from build123d import *

# Parameters (mm, degrees)
SKETCH1_W           = 43
SKETCH1_H           = 13
SKETCH1_R           = 1.2
SKETCH1_R_2         = 0.5
SKETCH1_W_2         = 1
SKETCH1_H_2         = 1
BOSS_EXTRUDE1_DEPTH = 1.1
SKETCH4_W           = 0.574829242
SKETCH4_H           = 0.46096735
CUT_EXTRUDE3_DEPTH  = 45.935620614
SKETCH2_R           = 0.75
CUT_EXTRUDE1_DEPTH  = 1.1
SKETCH5_R           = 0.85
CUT_EXTRUDE4_DEPTH  = 45.935620614
SKETCH3_W           = 2
SKETCH3_H           = 2
BOSS_EXTRUDE4_DEPTH = 0.75
SKETCH8_W           = 1.866359835
SKETCH8_H           = 4.750734125
SKETCH8_W_2         = 2.60606497
SKETCH8_H_2         = 3.913085661
SKETCH8_W_3         = 1.175159236
SKETCH8_H_3         = 2.413325778
SKETCH8_W_4         = 2.289773106
SKETCH8_H_4         = 4.453019048
SKETCH8_W_5         = 2.5
SKETCH8_H_5         = 3.5
BOSS_EXTRUDE5_DEPTH = 1.6
SKETCH9_W           = 2
SKETCH9_H           = 3
SKETCH9_W_2         = 2.013067154
BOSS_EXTRUDE6_DEPTH = 1
SKETCH11_R          = 1
BOSS_EXTRUDE7_DEPTH = 1.4


with BuildPart() as part:
    # Sketch1 → Boss-Extrude1 (new body)
    with BuildSketch(Plane(origin=(0, 0, 0), x_dir=(1, 0, 0), z_dir=(0, 1, 0))):
        with Locations((21.5, 6.5)):
            Rectangle(SKETCH1_W, SKETCH1_H)
        with Locations(Location((2, 7, 0), (0, 0, 270))):
            Circle(SKETCH1_R, mode=Mode.SUBTRACT)
        with Locations(Location((31, 7, 0), (0, 0, 270))):
            Circle(SKETCH1_R, mode=Mode.SUBTRACT)
        with Locations(Location((38.6, 7, 0), (0, 0, 270))):
            Circle(SKETCH1_R_2, mode=Mode.SUBTRACT)
        with Locations(Location((41.412673615, 7, 0), (0, 0, 270))):
            Circle(SKETCH1_R_2, mode=Mode.SUBTRACT)
        with Locations(Location((38.6, 9.7, 0), (0, 0, 270))):
            Circle(SKETCH1_R_2, mode=Mode.SUBTRACT)
        with Locations(Location((41.5, 9.7, 0), (0, 0, 270))):
            Circle(SKETCH1_R_2, mode=Mode.SUBTRACT)
        with Locations((38.6, 4.4)):
            Rectangle(SKETCH1_W_2, SKETCH1_H_2, mode=Mode.SUBTRACT)
        with Locations((41.5, 4.4)):
            Rectangle(SKETCH1_W_2, SKETCH1_H_2, mode=Mode.SUBTRACT)
    extrude(amount=BOSS_EXTRUDE1_DEPTH)

    # Sketch4 → Cut-Extrude3 (cut, through all)
    with BuildSketch(Plane(origin=(0, 1.1, 0), x_dir=(1, 0, 0), z_dir=(0, 1, 0))):
        with Locations((10.5, 6.769516325)):
            Rectangle(SKETCH4_W, SKETCH4_H)
    extrude(amount=-CUT_EXTRUDE3_DEPTH, mode=Mode.SUBTRACT)

    # Sketch2 → Cut-Extrude1 (cut)
    with BuildSketch(Plane(origin=(0, 1.1, 0), x_dir=(1, 0, 0), z_dir=(0, 1, 0))):
        with Locations(Location((6, 6.769516325, 0), (0, 0, 270))):
            Circle(SKETCH2_R)
    extrude(amount=-CUT_EXTRUDE1_DEPTH, mode=Mode.SUBTRACT)

    # Sketch5 → Cut-Extrude4 (cut, through all)
    with BuildSketch(Plane(origin=(0, 1.1, 0), x_dir=(1, 0, 0), z_dir=(0, 1, 0))):
        with Locations(Location((14, 6.769516325, 0), (0, 0, 270))):
            Circle(SKETCH5_R)
        with Locations(Location((17, 6.769516325, 0), (0, 0, 270))):
            Circle(SKETCH5_R)
    extrude(amount=-CUT_EXTRUDE4_DEPTH, mode=Mode.SUBTRACT)

    # Sketch3 → Boss-Extrude4 (add)
    with BuildSketch(Plane(origin=(0, 1.1, 0), x_dir=(1, 0, 0), z_dir=(0, 1, 0))):
        with Locations((10.5, 7)):
            Rectangle(SKETCH3_W, SKETCH3_H)
    extrude(amount=BOSS_EXTRUDE4_DEPTH)

    # Sketch8 → Boss-Extrude5 (add)
    with BuildSketch(Plane(origin=(0, 1.1, 0), x_dir=(1, 0, 0), z_dir=(0, 1, 0))):
        with Locations((5.784401845, 2.849545168)):
            Rectangle(SKETCH8_W, SKETCH8_H)
        with Locations((15.75, 2.849545168)):
            Rectangle(SKETCH8_W_2, SKETCH8_H_2)
        with Locations((20.25, 2.849545168)):
            Rectangle(SKETCH8_W_3, SKETCH8_H_3)
        with Locations((27.995132783, 2.574921462)):
            Rectangle(SKETCH8_W_4, SKETCH8_H_4)
        with Locations((14, 6.769516325)):
            Rectangle(SKETCH8_W_5, SKETCH8_H_5)
    extrude(amount=BOSS_EXTRUDE5_DEPTH)

    # Sketch9 → Boss-Extrude6 (add)
    with BuildSketch(Plane(origin=(0, 1.1, 0), x_dir=(1, 0, 0), z_dir=(0, 1, 0))):
        with Locations((35, 2)):
            Rectangle(SKETCH9_W, SKETCH9_H)
        with Locations((34.5, 11)):
            Rectangle(SKETCH9_W_2, SKETCH9_H)
        with Locations((30.5, 11)):
            Rectangle(SKETCH9_W, SKETCH9_H)
    extrude(amount=BOSS_EXTRUDE6_DEPTH)

    # Sketch11 → Boss-Extrude7 (add)
    with BuildSketch(Plane(origin=(0, 1.1, 0), x_dir=(1, 0, 0), z_dir=(0, 1, 0))):
        with Locations((14, 6.769516325)):
            Circle(SKETCH11_R)
    extrude(amount=BOSS_EXTRUDE7_DEPTH)


solid = part.part
Check sheet for the modelled part. Datum: model origin and axes. Units: mm. A direction names the side the tool comes from. Round coordinates to 2 decimals unless told otherwise and drop trailing zeros. Loops run counter-clockwise (first coordinate to the right, second up) from the corner with the lowest first, then second, coordinate; pieces in that order, holes last.
1. Gauge pin test, flat ends, axial feed: pin 1 Ø1 at (x, z) = (31.5, -11.5) entering from +Y; pin 2 Ø0.5 at (x, y) = (31, 1.5) entering from -Z; pin 3 Ø0.8 at (y, z) = (2, -11) entering from -X. Record the tip position at first contact, or that the pin passes through.
2. Sectioned sample at D-D on x = 31. Record the boundary of the cut face in (y, z), and give its area (3 significant figures).
3. Set-up check for faces 1 (the flat face through (20, 2, -1.643)), 2 (the cylindrical face through (14.843, 0.558, -6.88)), 3 (the flat face through (12.75, 2, -7)), 4 (the flat face through (34.5, 1.6, -12.5)), 5 (the flat face through (6, 2, -0.474)): record each of +Z, -Z, +X, -X, +Y, -Y from which the full face is reachable in a straight line by a thin tool's end or side.
4. Sectioned sample at C-C on z = -11.75. Record the boundary of the cut face in (x, y).
5. Sectioned sample at A-A on x = 38.6. Record the boundary of the cut face in (y, z).
6. Mould release check, pull along Z, two halves, no side actions. Record for faces 6 (the flat face through (34, 2.1, -11)), 7 (the flat face through (30.5, 1.6, -9.5)), 8 (the cylindrical face through (39.096, 0.542, -9.765)): released by +Z, released by -Z, zero draft, split by the parting line, or undercut.
7. Scan lines: probe 1 along X at (y, z) = (0.7, -9.7); probe 2 along Z at (x, y) = (41.5, 0.35); probe 3 along X at (y, z) = (2.4, -2). Record each from-to range of solid material in increasing order.
8. Sectioned sample at B-B on x = 2. Record the boundary of the cut face in (y, z).
Recorded:
1. pin 1: stops at y = 2.1
1. pin 2: stops at z = -12.5
1. pin 3: stops at x = 29.5
2. outline: (0, -13) - (1.1, -13) - (1.1, -12.5) - (2.1, -12.5) - (2.1, -9.5) - (1.1, -9.5) - (1.1, -8.2) - (0, -8.2) - close; (0, -5.8) - (1.1, -5.8) - (1.1, 0) - (0, 0) - close
2. area: 14.7 mm2
3. face 1: +Z, +Y
3. face 2: -Y
3. face 3: +Z, -Z, +Y
3. face 4: -Z, +X, -X, +Y
3. face 5: +Z, -X, +Y
4. outline: (0, 0) - (43, 0) - (43, 1.1) - (35.51, 1.1) - (35.51, 2.1) - (33.49, 2.1) - (33.49, 1.1) - (31.5, 1.1) - (31.5, 2.1) - (29.5, 2.1) - (29.5, 1.1) - (0, 1.1) - close
5. outline: (0, -13) - (1.1, -13) - (1.1, -10.2) - (0, -10.2) - close; (0, -9.2) - (1.1, -9.2) - (1.1, -7.5) - (0, -7.5) - close; (0, -6.5) - (1.1, -6.5) - (1.1, -4.9) - (0, -4.9) - close; (0, -3.9) - (1.1, -3.9) - (1.1, 0) - (0, 0) - close
6. face 6: zero draft
6. face 7: released by +Z
6. face 8: undercut
7. probe 1: x = 0 to 38.1, 39.1 to 41, 42 to 43
7. probe 2: z = -13 to -10.2, -9.2 to -7.49, -6.51 to -4.9, -3.9 to 0
7. probe 3: x = 4.85 to 6.72, 14.45 to 17.05, 19.66 to 20.84, 26.85 to 29.14
8. outline: (0, -13) - (1.1, -13) - (1.1, -8.2) - (0, -8.2) - close; (0, -5.8) - (1.1, -5.8) - (1.1, 0) - (0, 0) - close
